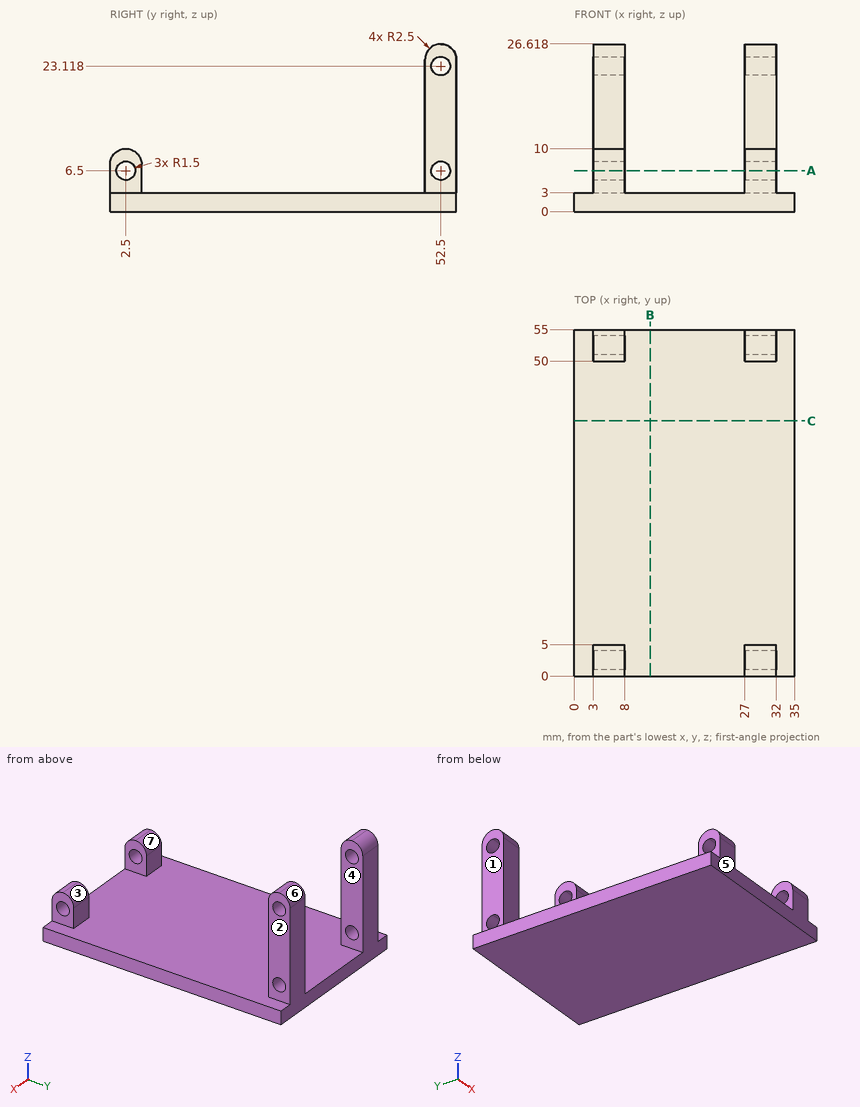
Geometry: see drawing. Coordinates: mm, zero at the bounding-box minimum. A direction names the side the tool comes from. Give positions to 0.01 mm unless a question says otherwise; leave off trailing zeros. Order: outer loops, then holes, each group sorted by start corner. A loop starts at its lowest first (then second) coordinate and runs counter-clockwise, first axis right, second up. Notation, with made-up numbers: M 37.25,59.5 L 50.25,59.5 A15 ccw 50.25,66.5 Z; hole C 7,6.5 d11. An arc over 180 degrees is marked long. Answer as a JSON object with one key per item and string values.
1. Cut plane A-A, the plane z = 6.5. State how many separate pieces and enclosed holes the cut face has.
Result sheet:
{"separate pieces": "8", "enclosed holes": "0"}
2. Pull-direction query (Y, two-part tool) for the marked faces 4, 5, 6 and 7; classes: +Y half, -Y half, draft (parallel to the pull), parting line (faces both ways), or undercut.
Result sheet:
{"face 4": "draft", "face 5": "-Y half", "face 6": "+Y half", "face 7": "undercut"}
3. First-contact query: P1, Ø2.5, axis at y = 52.5, z = 15, coming from the +X side; P2, Ø2.5, axis at y = 53.5, z = 12, coming from the -X side; P3, Ø2, axis at x = 6.5, y = 9, coming from the -Z side; P4, Ø5.5, axis at x = 28.5, z = 13.5, coming from the -Y side. Flat tips, straight axial feed; report the tip coordinate or a pass-through.
Result sheet:
{"P1": "x = 32", "P2": "x = 3", "P3": "z = 0", "P4": "y = 50"}
4. Cut plane C-C, the plane y = 40.5. Output: boundary loops of the cut face in (x, z).
Result sheet:
{"outline": "M 0,0 L 35,0 L 35,3 L 0,3 Z"}
5. Reachability of the marked faces 1, 2 and 3 from +Z, -Z, +X, -X, +Y, -Y: full face, straight path, thin tool, end or side. Return the list, or none.
Result sheet:
{"face 1": "+Z, -X, +Y, -Y", "face 2": "+Z, +X, +Y, -Y", "face 3": "+Z, +X, -X"}
6. Ray query, line 1 (Z direction, x = 9.5, y = 25.5); line 2 (Z direction, x = 7.5, y = 3.5); line 3 (Y direction, x = 28, z = 19.75). Return the intervals inside material, ascending. Write a range as [from, to].
Result sheet:
{"line 1": "[0, 3]", "line 2": "[0, 5.38], [7.62, 9.79]", "line 3": "[50, 55]"}
7. Cut plane B-B, the plane x = 12. Output: boundary loops of the cut face in (y, z), and give its area (3 significant figures).
Result sheet:
{"outline": "M 0,0 L 55,0 L 55,3 L 0,3 Z", "area": "165 mm²"}
